```python
from build123d import *

# Parameters (mm, degrees)
SKETCH1_W           = 80
SKETCH1_H           = 50
BOSS_EXTRUDE1_DEPTH = 5
SKETCH2_R           = 7.9
BOSS_EXTRUDE2_DEPTH = 5
SKETCH3_W           = 4.15
SKETCH3_H           = 50
BOSS_EXTRUDE3_DEPTH = 10
FILLET1_R           = 2
FILLET2_R           = 2


with BuildPart() as part:
    # Sketch1 → Boss-Extrude1 (new body)
    with BuildSketch(Plane(origin=(0, 0, 0), x_dir=(1, 0, 0), z_dir=(0, 1, 0))):
        Rectangle(SKETCH1_W, SKETCH1_H)
    extrude(amount=BOSS_EXTRUDE1_DEPTH)

    # Sketch2 → Boss-Extrude2 (add)
    with BuildSketch(Plane.XZ):
        with Locations(Location((-20.9, 0, 0), (0, 0, 270))):
            Circle(SKETCH2_R)
        with Locations(Location((20.9, 0, 0), (0, 0, 270))):
            Circle(SKETCH2_R)
    extrude(amount=BOSS_EXTRUDE2_DEPTH)

    # Sketch3 → Boss-Extrude3 (add)
    with BuildSketch(Plane(origin=(0, 5, 0), x_dir=(1, 0, 0), z_dir=(0, 1, 0))):
        with Locations((-37.925, 0)):
            Rectangle(SKETCH3_W, SKETCH3_H)
        with Locations((37.925, 0)):
            Rectangle(SKETCH3_W, SKETCH3_H)
    extrude(amount=BOSS_EXTRUDE3_DEPTH)

    # Fillet1
    fillet1_edges = [part.edges().sort_by_distance(p)[0] for p in [
        (-20.9, -5, 7.9),
        (20.9, -5, 7.9),
    ]]
    fillet(fillet1_edges, radius=FILLET1_R)

    # Fillet2
    fillet2_edges = [part.edges().sort_by_distance(p)[0] for p in [
        (0, 5, 25),
        (-35.85, 10, 25),
        (-35.85, 10, -25),
        (-37.925, 15, 25),
        (-35.85, 15, 0),
        (-37.925, 15, -25),
        (-40, 15, 0),
        (0, 5, -25),
        (35.85, 15, 0),
        (35.85, 10, -25),
        (35.85, 10, 25),
        (37.925, 15, 25),
        (40, 15, 0),
        (37.925, 15, -25),
        (0, 0, 25),
        (-40, 0, 0),
        (0, 0, -25),
        (40, 0, 0),
        (40, 7.5, 25),
        (-40, 7.5, 25),
        (-40, 7.5, -25),
        (40, 7.5, -25),
    ]]
    fillet(fillet2_edges, radius=FILLET2_R)


solid = part.part
```
Build history of the part. All positions in model axes, mm. A direction names the side the tool comes from. Coordinates: 2 decimals unless noted, no trailing zeros. Write each loop counter-clockwise with the first axis right and the second up, starting at its lowest first coordinate (ties: lowest second). Pieces come first, ordered by that corner, then holes.
1. Band-saw the part on C-C, the plane x = -20.9. Give the cut face in (y, z), and give its area (3 significant figures).
Answer block:
outline: (-5, -5.9) arc R2 ccw to (-3, -7.9) - (0, -7.9) - (0, -23) arc R2 ccw to (2, -25) - (3, -25) arc R2 ccw to (5, -23) - (5, 23) arc R2 ccw to (3, 25) - (2, 25) arc R2 ccw to (0, 23) - (0, 7.9) - (-3, 7.9) arc R2 ccw to (-5, 5.9) - close
area: 324 mm2
2. Pull direction X, two halves, no side cores. Call faces 4 (the cylindrical face through (39.4, 7.42, -24.43)), 5 (the flat face through (-1, 0, 0)), 6 (the cylindrical face through (-39.43, 7.58, 24.4)): released by +X, released by -X, zero draft, split by the parting line, or undercut.
Answer block:
face 4: released by +X
face 5: undercut
face 6: released by -X
3. Drill centre lines: probe 1 along X at (y, z) = (8.25, -2); probe 2 along X at (y, z) = (-0.75, 0); probe 3 along Z at (x, y) = (-4, 3.25). Where is each one in solid material? Low to high.
Answer block:
probe 1: x = -40 to -35.85, 35.85 to 40
probe 2: x = -28.8 to -13, 13 to 28.8
probe 3: z = -24.98 to 24.98
4. Band-saw the part on A-A, the plane z = 0. Give the cut face in (x, y), and give its area (3 significant figures).
Answer block:
outline: (-40, 2) arc R2 ccw to (-38, 0) - (-28.8, 0) - (-28.8, -3) arc R2 ccw to (-26.8, -5) - (-15, -5) arc R2 ccw to (-13, -3) - (-13, 0) - (13, 0) - (13, -3) arc R2 ccw to (15, -5) - (26.8, -5) arc R2 ccw to (28.8, -3) - (28.8, 0) - (38, 0) arc R2 ccw to (40, 2) - (40, 13) arc R2 ccw to (38, 15) - (37.85, 15) arc R2 ccw to (35.85, 13) - (35.85, 5) - (-35.85, 5) - (-35.85, 13) arc R2 ccw to (-37.85, 15) - (-38, 15) arc R2 ccw to (-40, 13) - close
area: 632 mm2
5. Band-saw the part on B-B, the plane x = 30. Give the cut face in (y, z).
Answer block:
outline: (0, -23) arc R2 ccw to (2, -25) - (3, -25) arc R2 ccw to (5, -23) - (5, 23) arc R2 ccw to (3, 25) - (2, 25) arc R2 ccw to (0, 23) - close
6. Band-saw the part on D-D, the plane z = 9. Give the cut face in (x, y).
Answer block:
outline: (-40, 2) arc R2 ccw to (-38, 0) - (38, 0) arc R2 ccw to (40, 2) - (40, 13) arc R2 ccw to (38, 15) - (37.85, 15) arc R2 ccw to (35.85, 13) - (35.85, 5) - (-35.85, 5) - (-35.85, 13) arc R2 ccw to (-37.85, 15) - (-38, 15) arc R2 ccw to (-40, 13) - close
7. 3-axis set-ups, long thin cutter, end or side, ignore diameter. For faces 1 (the flat face through (-0.2, 2.6, 25)), 2 (the flat face through (-35.85, 9, 0)), 3 (the cylindrical face through (-28.612, -1.479, 1.713)): which of +Z, -Z, +X, -X, +Y, -Y reach the whole face in a straight line?
Answer block:
face 1: +Z, +X, -X, +Y, -Y
face 2: +Z, -Z, +Y
face 3: -Y
8. Drop flat-ended pins along their axis: pin 1 (14 mm diameter, centred on x = -11.5, z = 6, fed in from +Y); pin 2 (8 mm diameter, centred on x = 1, y = -1, fed in from -Z); pin 3 (4 mm diameter, centred on x = -14.5, z = 5.5, fed in from -Y); pin 4 (1.5 mm diameter, centred on x = 0.5, y = 6, fed in from -Z). Give the stop position or say it passes through.
Answer block:
pin 1: stops at y = 5
pin 2: stops at z = -25
pin 3: stops at y = -4.93
pin 4: passes through
